Build history of the part. All positions in model axes, mm. Face numbers are marked on the shaded views. A direction names the side the tool comes from. Round coordinates to 2 decimals unless told otherwise and drop trailing zeros. Order: outer loops, then holes, each group sorted by start corner. A loop starts at its lowest first (then second) coordinate and runs counter-clockwise, first axis right, second up. Notation, with made-up numbers: M -24.75,-13 L 21.25,-13 A12 ccw 21.25,3 Z; hole C 33,12.5 d10. An arc over 180 degrees is marked long. One line per question, with ' | ' between items. Start each with the question number.
from build123d import *

# Parameters (mm, degrees)
SKETCH_1_W          = 7
SKETCH_1_H          = 14
SKETCH_1_W_2        = 20
SKETCH_1_H_2        = 7
EXTRUDE_1_DEPTH     = 10
SKETCH_2_R          = 3.65
CUT_EXTRUDE_1_DEPTH = 4.1
CUT_EXTRUDE_3_REACH = 28
SKETCH_4_W          = 7.3
SKETCH_4_H          = 7.3
CUT_EXTRUDE_2_REACH = 4.9
SKETCH_3_R          = 2.25


with BuildPart() as part:
    # 草圖1 → 填料-伸長1 (new body, symmetric)
    with BuildSketch(Plane.XY):
        with Locations((3.5, 14)):
            Rectangle(SKETCH_1_W, SKETCH_1_H)
        with Locations((10, 3.5)):
            Rectangle(SKETCH_1_W_2, SKETCH_1_H_2)
        Polygon((0, 26), (0, 21), (7, 21), (15, 21), (15, 26), align=None)
    extrude(amount=EXTRUDE_1_DEPTH, both=True)

    # 草圖2 → 除料-伸長1 (cut)
    with BuildSketch(Plane(origin=(0, 7, 0), x_dir=(1, 0, 0), z_dir=(0, 1, 0))):
        with Locations((12, 0)):
            Circle(SKETCH_2_R)
    extrude(amount=-CUT_EXTRUDE_1_DEPTH, mode=Mode.SUBTRACT)

    # 草圖4 → 除料-伸長3 (cut, up to next)
    with BuildSketch(Plane(origin=(0, 26, 0), x_dir=(1, 0, 0), z_dir=(0, 1, 0)), mode=Mode.PRIVATE) as cut_extrude_3_sk1:
        with Locations((12, 0)):
            Rectangle(SKETCH_4_W, SKETCH_4_H)
    cut_extrude_3_tool1 = extrude(cut_extrude_3_sk1.sketch, amount=-CUT_EXTRUDE_3_REACH, mode=Mode.PRIVATE) & part.part
    add(cut_extrude_3_tool1.solids().sort_by_distance((12, 26, 0))[0], mode=Mode.SUBTRACT)

    # 草圖3 → 除料-伸長2 (cut, up to next)
    with BuildSketch(Plane(origin=(0, 2.9, 0), x_dir=(1, 0, 0), z_dir=(0, 1, 0)), mode=Mode.PRIVATE) as cut_extrude_2_sk1:
        with Locations((12, 0)):
            Circle(SKETCH_3_R)
    cut_extrude_2_tool1 = extrude(cut_extrude_2_sk1.sketch, amount=-CUT_EXTRUDE_2_REACH, mode=Mode.PRIVATE) & part.part
    add(cut_extrude_2_tool1.solids().sort_by_distance((12, 2.9, 0))[0], mode=Mode.SUBTRACT)


solid = part.part
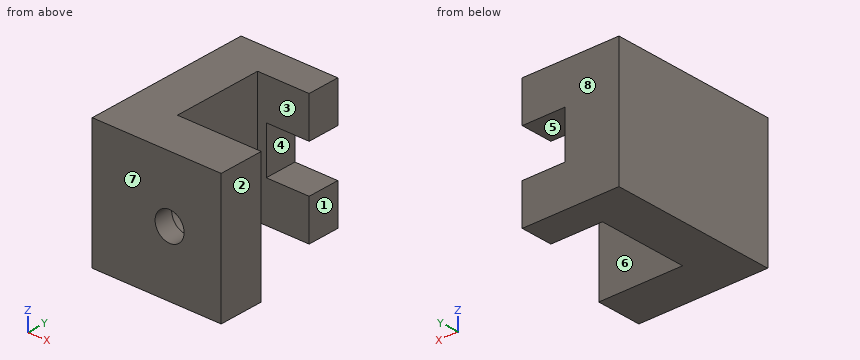
Item 1: Cut at A-A on x = 12. Write the cut outline in (y, z).
Item 2: Two-plate mould, pull along Y, no slides. Class the marked faces 5, 6, 7 and 8: +Y half, -Y half, draft (parallel to the pull), parting line (faces both ways), or undercut.
Item 3: Flat gauge pins, fed straight in: pin 1 (2.5 mm diameter, centred on y = 24, z = 1, fed in from +X); pin 2 (6 mm diameter, centred on y = 22, z = -2.5, fed in from +X); pin 3 (7 mm diameter, centred on y = 12, z = 3, fed in from +X); pin 4 (2 mm diameter, centred on x = 12, z = 1, fed in from +Y). Where does each tip first touch, or does it go through?
Item 4: Wall check: line 1 along X through (y, z) = (5.2, 0); line 2 along Y through (x, z) = (10.75, 5.5); line 3 along Z through (x, y) = (12, 1.3). Give the ranges that are in metal, low to high. Write a range as [from, to].
Item 5: Cut at C-C on z = 8.75. Write the cut outline in (x, y), then the cut area to 3 significant figures.
Item 6: Cut at B-B on z = 0. Write the cut outline in (x, y), then the cut area to 3 significant figures.
Item 7: Cut at D-D on y = 17.5. Write the cut outline in (x, z).
Item 8: Tool access for the marked faces 1, 2, 3 and 4: list every direction of +Z, -Z, +X, -X, +Y, -Y with a clear straight run to the whole face (end or side of a thin tool).
Results found:
1) outline: M 0,-10 L 7,-10 L 7,-3.65 L 2.9,-3.65 L 2.9,-2.25 L 0,-2.25 Z; M 0,2.25 L 2.9,2.25 L 2.9,3.65 L 7,3.65 L 7,10 L 0,10 Z; M 21,-10 L 26,-10 L 26,-3.65 L 21,-3.65 Z; M 21,3.65 L 26,3.65 L 26,10 L 21,10 Z
2) face 5: draft | face 6: undercut | face 7: -Y half | face 8: +Y half
3) pin 1: stops at x = 8.35 | pin 2: stops at x = 15 | pin 3: stops at x = 7 | pin 4: passes through
4) line 1: x = [0, 8.35], [15.65, 20] | line 2: y = [0, 7], [21, 26] | line 3: z = [-10, -2.25], [2.25, 10]
5) outline: M 0,0 L 20,0 L 20,7 L 7,7 L 7,21 L 15,21 L 15,26 L 0,26 Z | area: 313 mm^2
6) outline: M 0,0 L 9.75,0 L 9.75,2.9 L 8.35,2.9 L 8.35,7 L 7,7 L 7,21 L 8.35,21 L 8.35,26 L 0,26 Z; M 14.25,0 L 20,0 L 20,7 L 15.65,7 L 15.65,2.9 L 14.25,2.9 Z | area: 237 mm^2
7) outline: M 0,-10 L 7,-10 L 7,10 L 0,10 Z
8) face 1: +Z, -Z, +X, +Y | face 2: +Z, -Z, +X, +Y, -Y | face 3: +Z, -Z, +X | face 4: +X, +Y
